Job drawing, mm, ordinate dimensions from the low corner. One solid piece. A direction names the side the tool comes from. Coordinates: 2 decimals unless noted, no trailing zeros. Order: outer loops, then holes, each group sorted by start corner. A loop starts at its lowest first (then second) coordinate and runs counter-clockwise, first axis right, second up. Notation, with made-up numbers: (52.5, 12) - (106.5, 12) arc R21 ccw to (106.5, 31) - close; hole circle Ø9 at (57.25, 83.25). An arc over 180 degrees is marked (long way). Return JSON: item names as keys, results as strings.
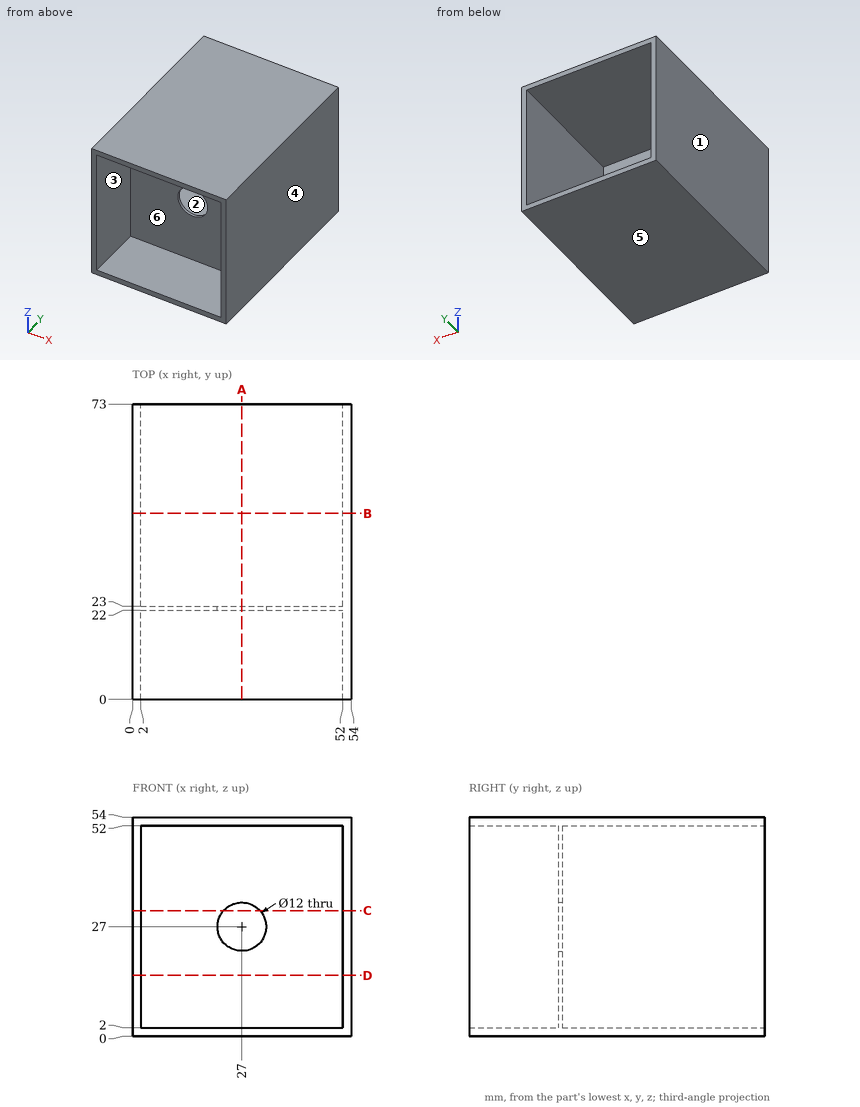
1. Cut at B-B on y = 46. Give the cut face in (x, z), plus the area to 3 significant figures.
Check values:
{"outline": "(0, 0) - (54, 0) - (54, 54) - (0, 54) - close; hole (2, 2) - (52, 2) - (52, 52) - (2, 52) - close", "area": "416 mm²"}
2. Cut at C-C on z = 31. Give the cut face in (x, y), plus the area to 3 significant figures.
Check values:
{"outline": "(0, 0) - (2, 0) - (2, 22) - (22.53, 22) - (22.53, 23) - (2, 23) - (2, 73) - (0, 73) - close; (31.47, 22) - (52, 22) - (52, 0) - (54, 0) - (54, 73) - (52, 73) - (52, 23) - (31.47, 23) - close", "area": "333 mm²"}
3. Drop flat-ended pins along their axis: pin 1 (25 mm diameter, centred on x = 24.5, z = 36.5, fed in from +Y); pin 2 (2 mm diameter, centred on x = 23, z = 36, fed in from -Y). Give the stop position or say it passes through.
Check values:
{"pin 1": "y = 23", "pin 2": "y = 22"}
4. Mould opens along Z. For the marked faces 4, 5 and 6 say: pulls with the +Z half, pulls with the -Z half, needs draft (parallel to the pull), parting line crosses it, or undercut.
Check values:
{"face 4": "needs draft", "face 5": "pulls with the -Z half", "face 6": "undercut"}
5. Probe L1, parallel to Z at x = 23.5, y = 65.5; L2, parallel to X at y = 22.85, z = 27. List the from-to ranges inside material, lowest first.
Check values:
{"L1": "0 to 2, 52 to 54", "L2": "0 to 21, 33 to 54"}
6. Tool access for the marked faces 1, 2 and 3: list every direction of +Z, -Z, +X, -X, +Y, -Y with a clear straight run to the whole face (end or side of a thin tool).
Check values:
{"face 1": "+Z, -Z, -X, +Y, -Y", "face 2": "+Y", "face 3": "-Y"}
7. Cut at D-D on z = 15. Give the cut face in (x, y).
Check values:
{"outline": "(0, 0) - (2, 0) - (2, 22) - (52, 22) - (52, 0) - (54, 0) - (54, 73) - (52, 73) - (52, 23) - (2, 23) - (2, 73) - (0, 73) - close"}
8. Cut at A-A on x = 27. Give the cut face in (y, z), plus the area to 3 significant figures.
Check values:
{"outline": "(0, 0) - (73, 0) - (73, 2) - (23, 2) - (23, 21) - (22, 21) - (22, 2) - (0, 2) - close; (0, 52) - (22, 52) - (22, 33) - (23, 33) - (23, 52) - (73, 52) - (73, 54) - (0, 54) - close", "area": "330 mm²"}
